```python
from build123d import *

# Parameters (mm, degrees)
F1_DEPTH = 3
F0_R     = 2.6
F0_W     = 13.2
F0_H     = 6
F0_W_2   = 2
F0_W_3   = 5.6
F0_H_2   = 8.5
F0_W_4   = 0.4
F0_H_3   = 2.75
F0_R_2   = 1.55
F2_DEPTH = 7.5
F3_DEPTH = 3.3


with BuildPart() as f1:
    # F0 (on Top) → F1 (new body)
    with BuildSketch(Plane.XY):
        Polygon((19.5, 13), (9.5, 13), (-3.7, 13), (-5.7, 13), (-18.9, 13), (-19.5, 13), (-19.5, -13), (-18.9, -13), (-5.7, -13), (-3.7, -13), (9.5, -13), (19.5, -13), (19.5, -7), (19.5, -4.25), (19.5, 4.25), (19.5, 7), align=None)
    extrude(amount=F1_DEPTH)

    # F0 (on Top) → F2 (join)
    with BuildSketch(Plane.XY):
        with BuildLine():
            Line((-18.9, 13), (-18.9, 19))
            Line((-18.9, 19), (-21.5, 19))
            ThreePointArc((-21.5, 19), (-24.3284271247, 17.8284271247), (-25.5, 15))
            Line((-25.5, 15), (-25.5, -15))
            ThreePointArc((-25.5, -15), (-24.3284271247, -17.8284271247), (-21.5, -19))
            Line((-21.5, -19), (-18.9, -19))
            Line((-18.9, -19), (-18.9, -13))
            Line((-18.9, -13), (-19.5, -13))
            Line((-19.5, -13), (-19.5, 13))
            Line((-19.5, 13), (-18.9, 13))
        make_face()
        with Locations((-21.8334523779, -15.3334523779)):
            Circle(F0_R, mode=Mode.SUBTRACT)
        with Locations((-21.8334523779, 15.3334523779)):
            Circle(F0_R, mode=Mode.SUBTRACT)
        with Locations((-12.3, -16)):
            Rectangle(F0_W, F0_H)
        with Locations((-4.7, -16)):
            Rectangle(F0_W_2, F0_H)
        with Locations((2.9, -16)):
            Rectangle(F0_W, F0_H)
        with BuildLine():
            Line((25.5, -15), (25.5, -7))
            Line((25.5, -7), (25.1, -7))
            Line((25.1, -7), (19.5, -7))
            Line((19.5, -7), (19.5, -13))
            Line((19.5, -13), (9.5, -13))
            Line((9.5, -13), (9.5, -19))
            Line((9.5, -19), (21.5, -19))
            ThreePointArc((21.5, -19), (24.3284271247, -17.8284271247), (25.5, -15))
        make_face()
        with Locations((21.8334523779, -15.3334523779)):
            Circle(F0_R, mode=Mode.SUBTRACT)
        with Locations((22.3, 0)):
            Rectangle(F0_W_3, F0_H_2)
        with Locations((25.3, -5.625)):
            Rectangle(F0_W_4, F0_H_3)
        with Locations((22.3, -5.625)):
            Rectangle(F0_W_3, F0_H_3)
        with Locations((25.3, 0)):
            Rectangle(F0_W_4, F0_H_2)
        with Locations((22.3, 5.625)):
            Rectangle(F0_W_3, F0_H_3)
        with Locations((25.3, 5.625)):
            Rectangle(F0_W_4, F0_H_3)
        with BuildLine():
            ThreePointArc((25.5, 15), (24.3284271247, 17.8284271247), (21.5, 19))
            Line((21.5, 19), (9.5, 19))
            Line((9.5, 19), (9.5, 13))
            Line((9.5, 13), (19.5, 13))
            Line((19.5, 13), (19.5, 7))
            Line((19.5, 7), (25.1, 7))
            Line((25.1, 7), (25.5, 7))
            Line((25.5, 7), (25.5, 15))
        make_face()
        with Locations((21.8334523779, 15.3334523779)):
            Circle(F0_R, mode=Mode.SUBTRACT)
        with Locations((2.9, 16)):
            Rectangle(F0_W, F0_H)
        with Locations((-4.7, 16)):
            Rectangle(F0_W_2, F0_H)
        with Locations((-12.3, 16)):
            Rectangle(F0_W, F0_H)
        with Locations((-21.8334523779, 15.3334523779)):
            Circle(F0_R)
        with Locations((-21.8334523779, 15.3334523779)):
            Circle(F0_R_2, mode=Mode.SUBTRACT)
        with Locations((-21.8334523779, -15.3334523779)):
            Circle(F0_R)
        with Locations((-21.8334523779, -15.3334523779)):
            Circle(F0_R_2, mode=Mode.SUBTRACT)
        with Locations((21.8334523779, -15.3334523779)):
            Circle(F0_R)
        with Locations((21.8334523779, -15.3334523779)):
            Circle(F0_R_2, mode=Mode.SUBTRACT)
        with Locations((21.8334523779, 15.3334523779)):
            Circle(F0_R)
        with Locations((21.8334523779, 15.3334523779)):
            Circle(F0_R_2, mode=Mode.SUBTRACT)
    extrude(amount=F2_DEPTH)

    # F0 (on Top) → F3 (cut)
    with BuildSketch(Plane.XY):
        with Locations((-21.8334523779, -15.3334523779)):
            Circle(F0_R)
        with Locations((-21.8334523779, -15.3334523779)):
            Circle(F0_R_2, mode=Mode.SUBTRACT)
        with Locations((21.8334523779, -15.3334523779)):
            Circle(F0_R)
        with Locations((21.8334523779, -15.3334523779)):
            Circle(F0_R_2, mode=Mode.SUBTRACT)
        with Locations((21.8334523779, 15.3334523779)):
            Circle(F0_R)
        with Locations((21.8334523779, 15.3334523779)):
            Circle(F0_R_2, mode=Mode.SUBTRACT)
        with Locations((-21.8334523779, 15.3334523779)):
            Circle(F0_R)
        with Locations((-21.8334523779, 15.3334523779)):
            Circle(F0_R_2, mode=Mode.SUBTRACT)
    extrude(amount=F3_DEPTH, mode=Mode.SUBTRACT)


solid = f1.part
```
The model under review builds one solid part; all positions refer to its coordinate system, in mm. A direction names the side the tool comes from. Round coordinates to 2 decimals unless told otherwise and drop trailing zeros. Write each loop counter-clockwise with the first axis right and the second up, starting at its lowest first coordinate (ties: lowest second). Pieces come first, ordered by that corner, then holes. Notation, with made-up numbers: M 74,84 L 95,84 A21 cw 95,97 Z; hole C 63,2 d4. An arc over 180 degrees is marked long. Use CSV: the item, a comma, the result in double quotes. Start each with the question number.
(1) Clearance check with flat-ended pins moving along their axes: P1, Ø2.5, axis at x = 22.5, y = -16, coming from the -Z side; P2, Ø1, axis at x = 1.5, y = -10.5, coming from the -Z side; P3, Ø3, axis at x = -21.83, y = -15.33, coming from the +Z side; P4, Ø10, axis at x = -12.5, y = 7.5, coming from the +Z side. State where each tip first meets the part, or that it passes through.
(2) We need section A-A, the plane x = -7. State the section outline as (y, z) points.
(3) The part is to be moulded in two halves that separate along X. For faces 4 (the face through (24.359, 17.797, 3.698)), 5 (the face through (23.265, -15.927, 5.371)), 6 (the face through (0, -19, 4)), say which applies: +X half, -X half, draft (parallel to the pull), parting line (faces both ways), or undercut.
(4) We need section B-B, the plane y = -12. State the section outline as (x, z) points, then the cut area to 3 significant figures.
(5) For line 1 along Y through (x, z) = (17, 5); line 2 along X through (y, z) = (-15, 6); line 3 along X through (y, z) = (16, 4.25), list the stretches that pass through material, from the lowest coordinate up.
(6) Tool access review of faces 1 (the face through (-21.1, -16.7, 5.4)), 2 (the face through (0, 0, 3)), 3 (the face through (-23.75, 17.09, 1.63)): name each direction out of +Z, -Z, +X, -X, +Y, -Y from which nothing blocks a thin tool from reaching the whole face with its end or side.
(7) We need section C-C, the plane z = 2.25. State the section outline as (x, y) points.
Findings:
1,P1,"z = 3.3"
1,P2,"z = 0"
1,P3,"through"
1,P4,"z = 3"
2,outline,"M -19,0 L 19,0 L 19,7.5 L 13,7.5 L 13,3 L -13,3 L -13,7.5 L -19,7.5 Z"
3,face 4,"+X half"
3,face 5,"undercut"
3,face 6,"draft"
4,outline,"M -25.5,0 L 25.5,0 L 25.5,7.5 L 19.5,7.5 L 19.5,3 L -19.5,3 L -19.5,7.5 L -25.5,7.5 Z"
4,area,"207 mm^2"
5,line 1,"-19 to -13, 13 to 19"
5,line 2,"-25.5 to -23.35, -20.32 to 20.32, 23.35 to 25.5"
5,line 3,"-25.37 to -23.23, -20.43 to 20.43, 23.23 to 25.37"
6,face 1,"+Z, -Z"
6,face 2,"+Z"
6,face 3,"-Z"
7,outline,"M -25.5,-15 A4 ccw -21.5,-19 L 21.5,-19 A4 ccw 25.5,-15 L 25.5,15 A4 ccw 21.5,19 L -21.5,19 A4 ccw -25.5,15 Z; hole C -21.83,-15.33 d5.2; hole C -21.83,15.33 d5.2; hole C 21.83,-15.33 d5.2; hole C 21.83,15.33 d5.2"
